from build123d import *

# Parameters (mm, degrees)
CHAMFER1_SIZE  = 0.50801365
EXTRUDE1_REACH = 57.499
CHAMFER2_SIZE  = 1.524


with BuildPart() as part:
    # Sketch1 → Revolve1 (revolve)
    with BuildSketch(Plane(origin=(0, 0, 0), x_dir=(1, 0, 0), z_dir=(0, 1, 0)), mode=Mode.PRIVATE) as revolve1_sk:
        Polygon((7.366, -27.7495), (7.366, 27.7495), (3.1623, 27.7495), (3.1623, 34.4805), (0, 34.4805), (0, -27.7495), align=None)
    revolve(revolve1_sk.sketch.rotate(Axis((0, 0, -34.4805), (0, 0, 1)), 180), axis=Axis((0, 0, -34.4805), (0, 0, 1)))  # turned: the seam where the file's is

    # Chamfer1
    chamfer1_edges = [part.edges().sort_by_distance(p)[0] for p in [
        (3.1623, 0, -34.4805),
    ]]
    chamfer(chamfer1_edges, length=CHAMFER1_SIZE)

    # Sketch2 → Extrude1 (cut, up to next)
    with BuildSketch(Plane(origin=(0, 0, -27.7495), x_dir=(-1, 0, 0), z_dir=(0, 0, -1)), mode=Mode.PRIVATE) as extrude1_sk1:
        with BuildLine():
            ThreePointArc((3.683, 6.379143124), (0, 7.366), (-3.683, 6.379143124))
            Line((-3.683, 6.379143124), (3.683, 6.379143124))
        make_face()
    extrude1_tool1 = extrude(extrude1_sk1.sketch, amount=-EXTRUDE1_REACH, mode=Mode.PRIVATE) & part.part
    add(extrude1_tool1.solids().sort_by_distance((0, 6.776244, -27.7495))[0], mode=Mode.SUBTRACT)
    # Sketch2 → Extrude1 (cut, up to next)
    with BuildSketch(Plane(origin=(0, 0, -27.7495), x_dir=(-1, 0, 0), z_dir=(0, 0, -1)), mode=Mode.PRIVATE) as extrude1_sk2:
        with BuildLine():
            ThreePointArc((7.366, 0), (6.379143124, 3.683), (3.683, 6.379143124))
            Line((3.683, 6.379143124), (7.366, 0))
        make_face()
    extrude1_tool2 = extrude(extrude1_sk2.sketch, amount=-EXTRUDE1_REACH, mode=Mode.PRIVATE) & part.part
    add(extrude1_tool2.solids().sort_by_distance((-5.868399, 3.388122, -27.7495))[0], mode=Mode.SUBTRACT)
    # Sketch2 → Extrude1 (cut, up to next)
    with BuildSketch(Plane(origin=(0, 0, -27.7495), x_dir=(-1, 0, 0), z_dir=(0, 0, -1)), mode=Mode.PRIVATE) as extrude1_sk3:
        with BuildLine():
            Line((7.366, 0), (3.683, -6.379143124))
            ThreePointArc((3.683, -6.379143124), (6.379143124, -3.683), (7.366, 0))
        make_face()
    extrude1_tool3 = extrude(extrude1_sk3.sketch, amount=-EXTRUDE1_REACH, mode=Mode.PRIVATE) & part.part
    add(extrude1_tool3.solids().sort_by_distance((-5.868399, -3.388122, -27.7495))[0], mode=Mode.SUBTRACT)
    # Sketch2 → Extrude1 (cut, up to next)
    with BuildSketch(Plane(origin=(0, 0, -27.7495), x_dir=(-1, 0, 0), z_dir=(0, 0, -1)), mode=Mode.PRIVATE) as extrude1_sk4:
        with BuildLine():
            Line((3.683, -6.379143124), (-3.683, -6.379143124))
            ThreePointArc((-3.683, -6.379143124), (0, -7.366), (3.683, -6.379143124))
        make_face()
    extrude1_tool4 = extrude(extrude1_sk4.sketch, amount=-EXTRUDE1_REACH, mode=Mode.PRIVATE) & part.part
    add(extrude1_tool4.solids().sort_by_distance((0, -6.776244, -27.7495))[0], mode=Mode.SUBTRACT)
    # Sketch2 → Extrude1 (cut, up to next)
    with BuildSketch(Plane(origin=(0, 0, -27.7495), x_dir=(-1, 0, 0), z_dir=(0, 0, -1)), mode=Mode.PRIVATE) as extrude1_sk5:
        with BuildLine():
            Line((-3.683, -6.379143124), (-7.366, 0))
            ThreePointArc((-7.366, 0), (-6.379143124, -3.683), (-3.683, -6.379143124))
        make_face()
    extrude1_tool5 = extrude(extrude1_sk5.sketch, amount=-EXTRUDE1_REACH, mode=Mode.PRIVATE) & part.part
    add(extrude1_tool5.solids().sort_by_distance((5.868399, -3.388122, -27.7495))[0], mode=Mode.SUBTRACT)
    # Sketch2 → Extrude1 (cut, up to next)
    with BuildSketch(Plane(origin=(0, 0, -27.7495), x_dir=(-1, 0, 0), z_dir=(0, 0, -1)), mode=Mode.PRIVATE) as extrude1_sk6:
        with BuildLine():
            ThreePointArc((-3.683, 6.379143124), (-6.379143124, 3.683), (-7.366, 0))
            Line((-7.366, 0), (-3.683, 6.379143124))
        make_face()
    extrude1_tool6 = extrude(extrude1_sk6.sketch, amount=-EXTRUDE1_REACH, mode=Mode.PRIVATE) & part.part
    add(extrude1_tool6.solids().sort_by_distance((5.868399, 3.388122, -27.7495))[0], mode=Mode.SUBTRACT)

    # Chamfer2
    chamfer2_edges = [part.edges().sort_by_distance(p)[0] for p in [
        (0, 6.379143124, -27.7495),
        (-5.5245, 3.189571562, -27.7495),
        (-5.5245, -3.189571562, -27.7495),
        (0, -6.379143124, -27.7495),
        (5.5245, -3.189571562, -27.7495),
        (5.5245, 3.189571562, -27.7495),
    ]]
    chamfer(chamfer2_edges, length=CHAMFER2_SIZE)


solid = part.part
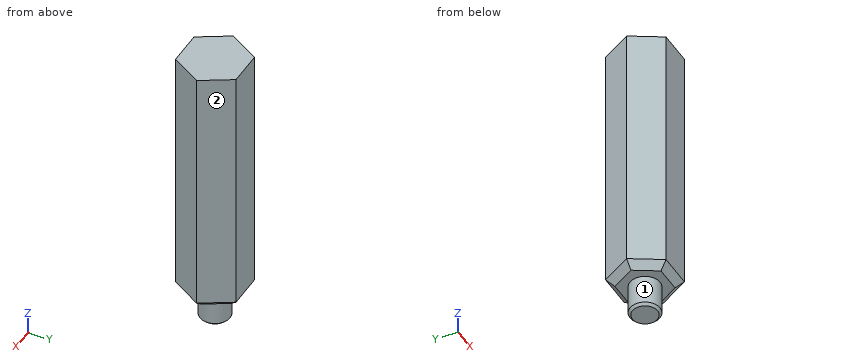
Read the model definition and answer for the solid it produces. Units are mm, in the model's axes. Face numbers are marked on the shaded views. A direction names the side the tool comes from. Coordinates: 2 decimals unless noted, no trailing zeros. Order: outer loops, then holes, each group sorted by start corner. A loop starts at its lowest first (then second) coordinate and runs counter-clockwise, first axis right, second up. Notation, with made-up numbers: (38.5, -26) -> (59.5, -26) arc R19 ccw to (59.5, 9) -> close; hole circle Ø11 at (-17, -12). An arc over 180 degrees is marked (long way). Answer as a JSON object with one key per item and string values.
1) A cutting plane is placed at C-C, the plane y = -3.75. Determine the outline of the cut face in (x, z).
Model answer:
{"outline": "(-5.2, -26.23) -> (-3.44, -27.75) -> (3.44, -27.75) -> (5.2, -26.23) -> (5.2, 27.75) -> (-5.2, 27.75) -> close"}
2) A tool of negligible diameter and unlimited length cuts with its end or side. For the marked faces 1 and 2, from which of +Z, -Z, +X, -X, +Y, -Y can it reach the whole face along a straight path? Write none if from no direction.
Model answer:
{"face 1": "-Z", "face 2": "+Z, -Z, +X, +Y"}
3) This flat-tipped pin is pushed along its axis until it touches: pin 1 (3 mm diameter, centred on x = -5, y = -4.5, fed in from -Z). Where does it stop, or does it pass through?
Model answer:
{"pin 1": "stops at z = -27.52"}
4) A cutting plane is placed at D-D, the plane z = -29. Determine the outline of the cut face in (x, y).
Model answer:
{"outline": "circle Ø6.32 at (0, 0)"}
5) A cutting plane is placed at B-B, the plane z = -9. Determine the outline of the cut face in (x, y), plus the area to 3 significant figures.
Model answer:
{"outline": "(-7.37, 0) -> (-3.68, -6.38) -> (3.68, -6.38) -> (7.37, 0) -> (3.68, 6.38) -> (-3.68, 6.38) -> close", "area": "141 mm²"}
6) Consider line 1 along Z through (x, y) = (1.75, 3.75); line 2 along Z through (x, y) = (-1.25, -5.5); line 3 along X through (y, z) = (-1, -7). Determine where each line is inside the solid, lowest interval first. Write a range as from..to.
Model answer:
{"line 1": "z = -27.75..27.75", "line 2": "z = -27.1..27.75", "line 3": "x = -6.79..6.79"}
7) A cutting plane is placed at A-A, the plane x = 0. Determine the outline of the cut face in (y, z), plus the area to 3 significant figures.
Model answer:
{"outline": "(-6.38, -26.23) -> (-4.86, -27.75) -> (-3.16, -27.75) -> (-3.16, -33.97) -> (-2.65, -34.48) -> (2.65, -34.48) -> (3.16, -33.97) -> (3.16, -27.75) -> (4.86, -27.75) -> (6.38, -26.23) -> (6.38, 27.75) -> (-6.38, 27.75) -> close", "area": "748 mm²"}
